Check sheet for the modelled part. Datum: model origin and axes. Units: mm. Give positions to 0.01 mm unless a question says otherwise; leave off trailing zeros. Write each loop counter-clockwise with the first axis right and the second up, starting at its lowest first coordinate (ties: lowest second). Pieces come first, ordered by that corner, then holes. Notation, with made-up numbers: M 63,13.5 L 121,13.5 A24 cw 121,23.5 Z; hole C 87.25,7 d1. An arc over 180 degrees is marked long. One line per item, written item: value. Start each with the question number.
from build123d import *

# Parameters (mm, degrees)
SKETCH_R        = 1
SKETCH_R_2      = 1.5
PAD_DEPTH       = 3
POCKET_DEPTH    = 1.25
SKETCH002_R     = 2.5
SKETCH002_R_2   = 1.5
PAD001_DEPTH    = 0.25
CHAMFER_SIZE    = 1
CHAMFER001_SIZE = 1.2


with BuildPart() as part:
    # Sketch → Pad (new body)
    with BuildSketch(Plane.YZ):
        Polygon((48.175426, 11.088705), (48.175426, -11.088705), (31.651763, -32.353395), (29.306974, -32.353395), (11.768704, -12.656963), (-4.783279, -12.656963), (-4.783279, 12.656963), (11.768704, 12.656963), (29.306974, 32.353395), (31.651763, 32.353395), align=None)
        with Locations((-2.283279, 10.156963)):
            Circle(SKETCH_R, mode=Mode.SUBTRACT)
        with Locations((23.920751, 3.649365)):
            Circle(SKETCH_R, mode=Mode.SUBTRACT)
        with Locations((30.428348, 29.853395)):
            Circle(SKETCH_R, mode=Mode.SUBTRACT)
        with Locations((-2.283279, -10.156963)):
            Circle(SKETCH_R, mode=Mode.SUBTRACT)
        with Locations((30.428348, -29.853395)):
            Circle(SKETCH_R, mode=Mode.SUBTRACT)
        with Locations((23.920751, -3.649365)):
            Circle(SKETCH_R, mode=Mode.SUBTRACT)
        with Locations((45, 10)):
            Circle(SKETCH_R_2, mode=Mode.SUBTRACT)
        with Locations((45, -10)):
            Circle(SKETCH_R_2, mode=Mode.SUBTRACT)
    extrude(amount=-PAD_DEPTH)

    # Sketch001 (on Face19 of Pad) → Pocket (cut)
    with BuildSketch(Plane.YZ):
        Polygon((43.354552, 12.85), (41.709103, 10), (43.354552, 7.15), (46.645448, 7.15), (48.175426, 7.15), (48.175426, 11.088705), (44.826178, 15.398932), align=None)
        Polygon((43.354552, -7.15), (41.709103, -10), (43.354552, -12.85), (44.826178, -15.398932), (48.175426, -11.088705), (48.175426, -7.15), (46.645448, -7.15), align=None)
    extrude(amount=-POCKET_DEPTH, mode=Mode.SUBTRACT)

    # Sketch002 (on Face5 of Pocket) → Pad001 (join)
    with BuildSketch(Plane(origin=(-3, 0, 0), x_dir=(0, 1, 0), z_dir=(-1, 0, 0))):
        with Locations((45, 10)):
            Circle(SKETCH002_R)
        with Locations((45, 10)):
            Circle(SKETCH002_R_2, mode=Mode.SUBTRACT)
        with Locations((45, -10)):
            Circle(SKETCH002_R)
        with Locations((45, -10)):
            Circle(SKETCH002_R_2, mode=Mode.SUBTRACT)
    extrude(amount=PAD001_DEPTH)

    # Chamfer
    chamfer_edges = [part.edges().sort_by_distance(p)[0] for p in [
        (-0.625, 44.826178, 15.398932),
        (-0.625, 48.175426, 7.15),
        (-0.625, 48.175426, -7.15),
        (-0.625, 44.826178, -15.398932),
        (-1.5, -4.783279, 12.656963),
        (-1.5, -4.783279, -12.656963),
    ]]
    chamfer(chamfer_edges, length=CHAMFER_SIZE)

    # Chamfer001
    chamfer001_edges = [part.edges().sort_by_distance(p)[0] for p in [
        (-3, 29.428348, 29.853395),
        (-3, 22.920751, 3.649365),
        (-3, 29.428348, -29.853395),
        (-3, -3.283279, -10.156963),
        (-3, -3.283279, 10.156963),
        (-3, 22.920751, -3.649365),
    ]]
    chamfer(chamfer001_edges, length=CHAMFER001_SIZE)


solid = part.part
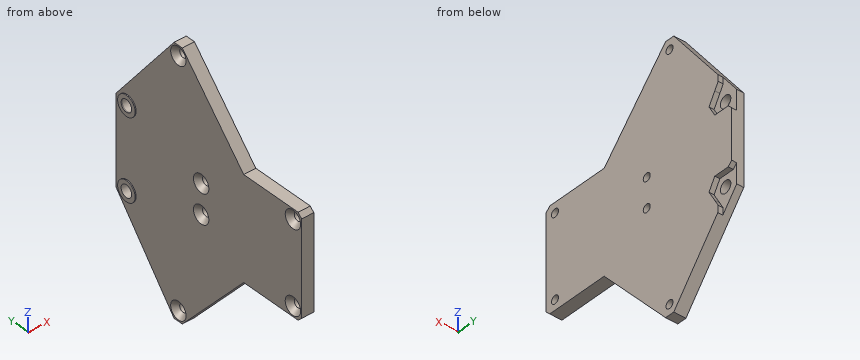
1) Material ranges on L1, parallel to Y at x = -3.05, z = 10; L2, parallel to Y at x = -2.5, z = 9.5; L3, parallel to Y at x = -2.7, z = 10.5, recorded low to high. Write a range as from..to.
2) Cross-section at C-C (y = 1). Record the boundary of the cut face in (x, z), plus the area to 3 significant figures.
3) Gauge pin test, flat ends, axial feed: pin 1 (3 mm diameter, centred on y = 30.43, z = 29.85, fed in from -X); pin 2 (1.5 mm diameter, centred on y = 13.5, z = -13, fed in from -X); pin 3 (1.2 mm diameter, centred on y = -2.28, z = -10.16, fed in from -X); pin 4 (5 mm diameter, centred on y = 45, z = 10, fed in from +X). Record the tip position at first contact, or that the pin passes through.
4) Cross-section at B-B (y = 45). Record the boundary of the cut face in (x, z), plus the area to 3 significant figures.
5) Cross-section at D-D (z = 25). Record the boundary of the cut face in (x, y).
6) Cross-section at A-A (x = -2.3). State how many separate pieces and enclosed holes the cut face has, plus the area to 3 significant figures.
Data:
1. L1: y = 42.5..43.5, 46.5..47.5
1. L2: y = -4.78..-3.85, -0.72..43.59, 46.41..48.18
1. L3: y = -4.78..-4.15, -0.41..43.59, 46.41..48.18
2. outline: M -3,-12.66 L 0,-12.66 L 0,12.66 L -3,12.66 Z
2. area: 75.9 mm2
3. pin 1: stops at x = -2.3
3. pin 2: stops at x = -3
3. pin 3: passes through
3. pin 4: stops at x = -1.25
4. outline: M -3.25,-12.5 L -3,-12.5 L -3,-15.18 L -1.25,-15.18 L -1.25,-11.5 L -3.25,-11.5 Z; M -3.25,-8.5 L -1.25,-8.5 L -1.25,-7.15 L 0,-7.15 L 0,7.15 L -1.25,7.15 L -1.25,8.5 L -3.25,8.5 L -3.25,7.5 L -3,7.5 L -3,-7.5 L -3.25,-7.5 Z; M -3.25,11.5 L -1.25,11.5 L -1.25,15.18 L -3,15.18 L -3,12.5 L -3.25,12.5 Z
4. area: 61.5 mm2
5. outline: M -3,22.76 L 0,22.76 L 0,37.37 L -3,37.37 Z
6. separate pieces: 1
6. enclosed holes: 8
6. area: 2,020 mm2
